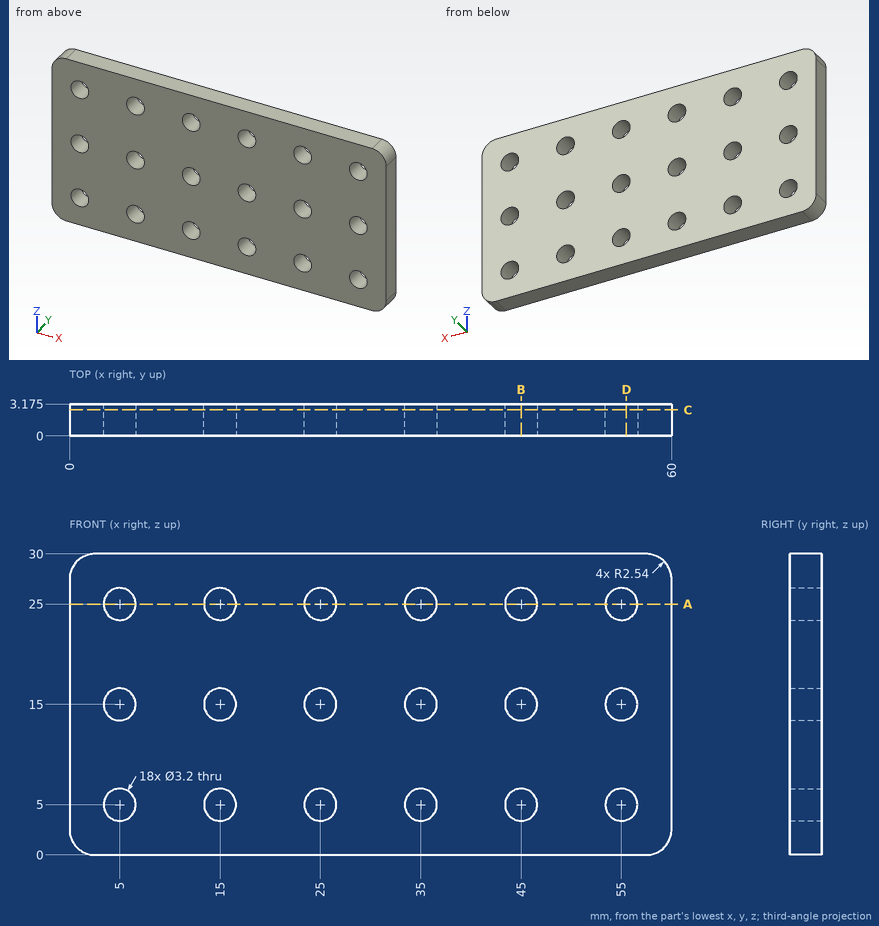
Geometry check sheet. Reference: drawing and pictorial views, mm from the part's lowest x, y, z. Coordinates: 2 decimals unless noted, no trailing zeros. Order: outer loops, then holes, each group sorted by start corner. A loop starts at its lowest first (then second) coordinate and runs counter-clockwise, first axis right, second up. Notation, with made-up numbers: (57.25, -25.5) - (104.25, -25.5) arc R11 ccw to (104.25, -14.5) - close; hole circle Ø7 at (24, -12). An arc over 180 degrees is marked (long way). One line per item, written item: value.
(1) Sectioned sample at D-D (x = 55.5). Enter the section's corners in (y, z) (3 decimals).
Data:
outline: (0, 0) - (3.175, 0) - (3.175, 3.48) - (0, 3.48) - close; (0, 6.52) - (3.175, 6.52) - (3.175, 13.48) - (0, 13.48) - close; (0, 16.52) - (3.175, 16.52) - (3.175, 23.48) - (0, 23.48) - close; (0, 26.52) - (3.175, 26.52) - (3.175, 30) - (0, 30) - close
(2) Sectioned sample at C-C (y = 2.6). Count the separate pieces of the cut face and the enclosed holes in it, and give its area (3 significant figures).
Data:
separate pieces: 1
enclosed holes: 18
area: 1,650 mm^2
(3) Sectioned sample at A-A (z = 25). Enter the section's corners in (x, y) (3 decimals), and give its area (3 significant figures).
Data:
outline: (0, 0) - (3.4, 0) - (3.4, 3.175) - (0, 3.175) - close; (6.6, 0) - (13.4, 0) - (13.4, 3.175) - (6.6, 3.175) - close; (16.6, 0) - (23.4, 0) - (23.4, 3.175) - (16.6, 3.175) - close; (26.6, 0) - (33.4, 0) - (33.4, 3.175) - (26.6, 3.175) - close; (36.6, 0) - (43.4, 0) - (43.4, 3.175) - (36.6, 3.175) - close; (46.6, 0) - (53.4, 0) - (53.4, 3.175) - (46.6, 3.175) - close; (56.6, 0) - (60, 0) - (60, 3.175) - (56.6, 3.175) - close
area: 130 mm^2
(4) Thickness scan on probe 1 along Z at (x, y) = (5, 1.1); probe 2 along Z at (x, y) = (14, 1.6). Record the ranges inside material, lowest first. Write a range as from..to.
Data:
probe 1: z = 0..3.4, 6.6..13.4, 16.6..23.4, 26.6..30
probe 2: z = 0..3.75, 6.25..13.75, 16.25..23.75, 26.25..30
(5) Sectioned sample at B-B (x = 45). Enter the section's corners in (y, z) (3 decimals), and give its area (3 significant figures).
Data:
outline: (0, 0) - (3.175, 0) - (3.175, 3.4) - (0, 3.4) - close; (0, 6.6) - (3.175, 6.6) - (3.175, 13.4) - (0, 13.4) - close; (0, 16.6) - (3.175, 16.6) - (3.175, 23.4) - (0, 23.4) - close; (0, 26.6) - (3.175, 26.6) - (3.175, 30) - (0, 30) - close
area: 64.8 mm^2
